Here's how the part is built. I have some questions about the finished solid (model axes, mm). Face numbers are marked on the shaded views. Round coordinates to 2 decimals unless told otherwise and drop trailing zeros. Write each loop counter-clockwise with the first axis right and the second up, starting at its lowest first coordinate (ties: lowest second). Pieces come first, ordered by that corner, then holes. Notation, with made-up numbers: (6, 46.5) -> (32, 46.5) arc R15 ccw to (32, 54.5) -> close; hole circle Ø3 at (36, 83). An arc over 180 degrees is marked (long way). Answer in a Markdown table with one row per item.
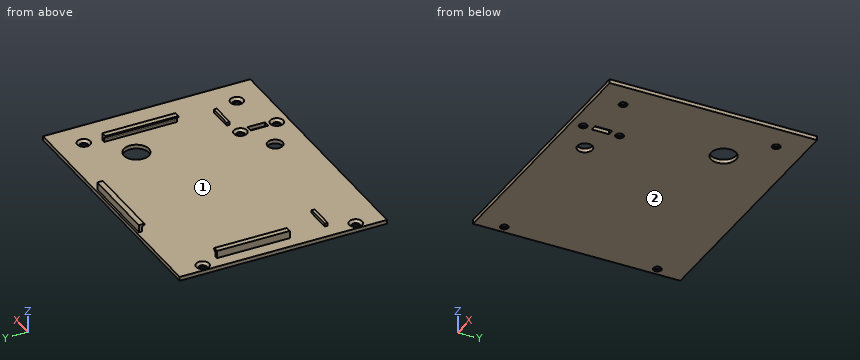
from build123d import *

# Parameters (mm, degrees)
F0_W      = 105.35
F0_H      = 82.6
F0_R      = 1.6
F3_DEPTH  = 1.6
F1_R      = 5
F4_DEPTH  = 1.601
F2_R      = 1.6
F2_R_2    = 3
F2_W      = 2.5
F2_H      = 7
F5_DEPTH  = 1.601
F7_START  = -36.1
F7_DEPTH  = 29
F9_START  = 33
F9_DEPTH  = 32
F1_W      = 10
F1_H      = 1.2
F10_DEPTH = 1.2
F11_SIZE  = 1


with BuildPart() as f3:
    # F0 (on Top) → F3 (new body)
    with BuildSketch(Plane.XY):
        with Locations((52.675, 41.3)):
            Rectangle(F0_W, F0_H)
        with Locations((3.2, 10.8)):
            Circle(F0_R, mode=Mode.SUBTRACT)
        with Locations((94.8, 10.8)):
            Circle(F0_R, mode=Mode.SUBTRACT)
        with Locations((3.2, 71.8)):
            Circle(F0_R, mode=Mode.SUBTRACT)
        with Locations((94.8, 71.8)):
            Circle(F0_R, mode=Mode.SUBTRACT)
    extrude(amount=-F3_DEPTH)

    # F1 (on face) → F4 (cut, through all)
    with BuildSketch(Plane.XY):
        with Locations((80.75, 58.1)):
            Circle(F1_R)
    extrude(amount=-F4_DEPTH, mode=Mode.SUBTRACT)

    # F2 (on face) → F5 (cut, through all)
    with BuildSketch(Plane.XY):
        with Locations((75.75, 4.75)):
            Circle(F2_R)
        with Locations((63, 12)):
            Circle(F2_R_2)
        with Locations((76.25, 12)):
            Rectangle(F2_W, F2_H)
        with Locations((75.75, 19.25)):
            Circle(F2_R)
    extrude(amount=-F5_DEPTH, mode=Mode.SUBTRACT)

    # F6 (on Front) → F7 (join)
    with BuildSketch(Plane.XZ.offset(F7_START)):
        with BuildLine():
            add(Edge.make_bspline(
                [(6.25, 0.9831411553), (6.1998556443, 0.4976120788), (6.25, 0.0696883488), (6.25, 0)],
                knots=[1.5113210061, 1.5113210061, 1.5113210061, 1.5113210061, 2.6925824036, 2.6925824036, 2.6925824036, 2.6925824036], degree=3))
            Line((6.25, 0), (6.25, 0.9831411553))
        make_face()
        with BuildLine():
            Line((5.05, 0), (6.25, 0))
            add(Edge.make_bspline(
                [(6.25, 0.9831411553), (6.1998556443, 0.4976120788), (6.25, 0.0696883488), (6.25, 0)],
                knots=[1.5113210061, 1.5113210061, 1.5113210061, 1.5113210061, 2.6925824036, 2.6925824036, 2.6925824036, 2.6925824036], degree=3))
            Line((6.25, 0.9831411553), (6.25, 3))
            Line((6.25, 3), (5.05, 3))
            Line((5.05, 3), (5.05, 0))
        make_face()
        with BuildLine():
            Line((6.25, 3), (6.25, 0.9831411553))
            add(Edge.make_bspline(
                [(7.25, 2.5), (6.5424729796, 2.3198194624), (6.3141553328, 1.6043332928), (6.25, 0.9831411553)],
                knots=[0, 0, 0, 0, 1.5113210061, 1.5113210061, 1.5113210061, 1.5113210061], degree=3))
            Line((7.25, 2.5), (7.25, 3))
            Line((7.25, 3), (6.25, 3))
        make_face()
        with BuildLine():
            Line((92.05, 0.9831411553), (92.05, 3))
            Line((92.05, 3), (91.05, 3))
            Line((91.05, 3), (91.05, 2.5))
            add(Edge.make_bspline(
                [(91.05, 2.5), (91.7575270204, 2.3198194624), (91.9858446672, 1.6043332928), (92.05, 0.9831411553)],
                knots=[0, 0, 0, 0, 1.5113210061, 1.5113210061, 1.5113210061, 1.5113210061], degree=3))
        make_face()
        with BuildLine():
            Line((93.25, 3), (92.05, 3))
            Line((92.05, 3), (92.05, 0.9831411553))
            add(Edge.make_bspline(
                [(92.05, 0.9831411553), (92.1001443557, 0.4976120788), (92.05, 0.0696883488), (92.05, 0)],
                knots=[1.5113210061, 1.5113210061, 1.5113210061, 1.5113210061, 2.6925824036, 2.6925824036, 2.6925824036, 2.6925824036], degree=3))
            Line((92.05, 0), (93.25, 0))
            Line((93.25, 0), (93.25, 3))
        make_face()
        with BuildLine():
            add(Edge.make_bspline(
                [(92.05, 0.9831411553), (92.1001443557, 0.4976120788), (92.05, 0.0696883488), (92.05, 0)],
                knots=[1.5113210061, 1.5113210061, 1.5113210061, 1.5113210061, 2.6925824036, 2.6925824036, 2.6925824036, 2.6925824036], degree=3))
            Line((92.05, 0.9831411553), (92.05, 0))
        make_face()
    extrude(amount=-F7_DEPTH)

    # F8 (on Right) → F9 (join)
    with BuildSketch(Plane.YZ.offset(F9_START)):
        with BuildLine():
            add(Edge.make_bspline(
                [(80.6190222502, 1.5), (80.7199138112, 0.9911874772), (80.6190222502, 0.2993458475), (80.6190222502, 0)],
                knots=[0.4926390921, 0.4926390921, 0.4926390921, 0.4926390921, 1, 1, 1, 1], degree=3))
            Line((80.6190222502, 0), (81.8190222502, 0))
            Line((81.8190222502, 0), (81.8190222502, 3))
            Line((81.8190222502, 3), (80.6190222502, 3))
            Line((80.6190222502, 3), (80.6190222502, 1.5))
        make_face()
        with BuildLine():
            Line((80.6190222502, 1.5), (80.6190222502, 0))
            add(Edge.make_bspline(
                [(80.6190222502, 1.5), (80.7199138112, 0.9911874772), (80.6190222502, 0.2993458475), (80.6190222502, 0)],
                knots=[0.4926390921, 0.4926390921, 0.4926390921, 0.4926390921, 1, 1, 1, 1], degree=3))
        make_face()
        with BuildLine():
            add(Edge.make_bspline(
                [(79.6190222502, 2.5), (80.2328512073, 2.3155356757), (80.5210582047, 1.9940485863), (80.6190222502, 1.5)],
                knots=[0, 0, 0, 0, 0.4926390921, 0.4926390921, 0.4926390921, 0.4926390921], degree=3))
            Line((80.6190222502, 1.5), (80.6190222502, 3))
            Line((80.6190222502, 3), (79.6190222502, 3))
            Line((79.6190222502, 3), (79.6190222502, 2.5))
        make_face()
    extrude(amount=F9_DEPTH)

    # F1 (on face) → F10 (join)
    with BuildSketch(Plane.XY):
        with Locations((11.25, 21)):
            Rectangle(F1_W, F1_H)
        with Locations((86.75, 21)):
            Rectangle(F1_W, F1_H)
    extrude(amount=F10_DEPTH)

    # F11
    f11_edges = [f3.edges().sort_by_distance(p)[0] for p in [
        (1.6, 71.8, 0),
        (93.2, 71.8, 0),
        (93.2, 10.8, 0),
        (74.15, 19.25, 0),
        (74.15, 4.75, 0),
        (1.6, 10.8, 0),
    ]]
    chamfer(f11_edges, length=F11_SIZE)


solid = f3.part
1) For pin 1 (0.6 mm diameter, centred on x = 11, z = 0.5, fed in from -Y); pin 2 (3 mm diameter, centred on x = 28.5, y = 71, fed in from +Z); pin 3 (1 mm diameter, centred on y = 21, z = 1, fed in from +X), each with a flat end and sliding along its axis, tell me the tip position at first contact or that it passes through.
Response:
| item | result |
|---|---|
| pin 1 | stops at y = 20.4 |
| pin 2 | stops at z = 0 |
| pin 3 | stops at x = 91.75 |
2) I need wall thicknesses on line 1 (Y direction, x = 3.2, z = -1.15); line 2 (X direction, y = 21, z = 1.05); line 3 (Z direction, x = 22.5, y = 36). Which ranges of each line are inside material? Lowest first, please. Write a range as [from, to].
Response:
| item | result |
|---|---|
| line 1 | y = [0, 9.2], [12.4, 70.2], [73.4, 82.6] |
| line 2 | x = [6.25, 16.25], [81.75, 91.75] |
| line 3 | z = [-1.6, 0] |
3) I want a section at A-A, the plane y = 4.75. List the corners of the cut face in (x, z) for me.
Response:
| item | result |
|---|---|
| outline | (0, -1.6) -> (74.15, -1.6) -> (74.15, -1) -> (73.15, 0) -> (0, 0) -> close; (77.35, -1.6) -> (105.35, -1.6) -> (105.35, 0) -> (78.35, 0) -> (77.35, -1) -> close |
4) We'd pull the mould along X, two halves only. Please class the marked faces 1 and 2: +X half, -X half, draft (parallel to the pull), parting line (faces both ways), or undercut.
Response:
| item | result |
|---|---|
| face 1 | undercut |
| face 2 | draft |
5) I want a section at B-B, the plane x = 26. List the corners of the cut face in (y, z) for me.
Response:
| item | result |
|---|---|
| outline | (0, -1.6) -> (82.6, -1.6) -> (82.6, 0) -> (0, 0) -> close |
